```python
from build123d import *

# Parameters (mm, degrees)
SKETCH1_W            = 93
SKETCH1_H            = 60
BOSS_EXTRUDE1_DEPTH  = 3
SKETCH2_W            = 3
SKETCH2_H            = 5
CUT_EXTRUDE1_DEPTH   = 3
SKETCH4_W            = 35
SKETCH4_H            = 3
BOSS_EXTRUDE2_DEPTH  = 45
FILLET1_R            = 5
SKETCH5_W            = 3
SKETCH5_H            = 5
CUT_EXTRUDE3_DEPTH   = 4
LPATTERN1_COUNT      = 4
LPATTERN1_PITCH      = 30
LPATTERN1_COUNT_DIR2 = 2
LPATTERN1_PITCH_DIR2 = 30
SKETCH6_R            = 2
CUT_EXTRUDE4_DEPTH   = 4
SKETCH7_W            = 3
SKETCH7_H            = 5
CUT_EXTRUDE5_DEPTH   = 4
SKETCH8_R            = 3
CUT_EXTRUDE6_DEPTH   = 4


with BuildPart() as part:
    # Sketch1 → Boss-Extrude1 (new body)
    with BuildSketch(Plane(origin=(0, 0, 0), x_dir=(1, 0, 0), z_dir=(0, 1, 0))):
        with Locations((46.5, 30)):
            Rectangle(SKETCH1_W, SKETCH1_H)
    extrude(amount=BOSS_EXTRUDE1_DEPTH)

    # Sketch2 → Cut-Extrude1 (cut)
    with BuildSketch(Plane(origin=(0, 3, 0), x_dir=(1, 0, 0), z_dir=(0, 1, 0))):
        with Locations((63.5, 12.5)):
            Rectangle(SKETCH2_W, SKETCH2_H)
        with Locations((47.5, 12.5)):
            Rectangle(SKETCH2_W, SKETCH2_H)
        with Locations((29.5, 12.5)):
            Rectangle(SKETCH2_W, SKETCH2_H)
        with Locations((6.5, 12.5)):
            Rectangle(SKETCH2_W, SKETCH2_H)
    cut_extrude1 = extrude(amount=-CUT_EXTRUDE1_DEPTH, mode=Mode.SUBTRACT)

    # Mirror1: Cut-Extrude1 across plane
    add(cut_extrude1.mirror(Plane.XY.offset(-30)), mode=Mode.SUBTRACT)

    # Sketch4 → Boss-Extrude2 (add)
    with BuildSketch(Plane(origin=(0, 0, -60), x_dir=(-1, 0, 0), z_dir=(0, 0, -1))):
        with Locations((-75.5, 1.5)):
            Rectangle(SKETCH4_W, SKETCH4_H)
    extrude(amount=BOSS_EXTRUDE2_DEPTH)

    # Fillet1
    fillet1_edges = [part.edges().sort_by_distance(p)[0] for p in [
        (58, 1.5, -60),
        (93, 1.5, -105),
        (58, 1.5, -105),
        (0, 1.5, -60),
        (93, 1.5, 0),
        (0, 1.5, 0),
    ]]
    fillet(fillet1_edges, radius=FILLET1_R)

    # Sketch5 → Cut-Extrude3 (cut, through all)
    with BuildSketch(Plane(origin=(0, 3, 0), x_dir=(1, 0, 0), z_dir=(0, 1, 0))):
        with Locations((86.5, 7.5)):
            Rectangle(SKETCH5_W, SKETCH5_H)
        with Locations((79.5, 7.5)):
            Rectangle(SKETCH5_W, SKETCH5_H)
    cut_extrude3 = extrude(amount=-CUT_EXTRUDE3_DEPTH, mode=Mode.SUBTRACT)

    # LPattern1: Cut-Extrude3 4 × 2
    with Locations(*[(j * LPATTERN1_PITCH_DIR2, 0, -i * LPATTERN1_PITCH) for i in range(LPATTERN1_COUNT) for j in range(LPATTERN1_COUNT_DIR2) if (i, j) != (0, 0)]):
        add(cut_extrude3, mode=Mode.SUBTRACT)

    # Sketch6 → Cut-Extrude4 (cut, through all)
    with BuildSketch(Plane(origin=(0, 3, 0), x_dir=(1, 0, 0), z_dir=(0, 1, 0))):
        with Locations((18, 14)):
            Circle(SKETCH6_R)
        with Locations((18, 46)):
            Circle(SKETCH6_R)
        with Locations((55.5, 50.5)):
            Circle(SKETCH6_R)
        with Locations((55.5, 9.5)):
            Circle(SKETCH6_R)
        with Locations((72, 9.5)):
            Circle(SKETCH6_R)
        with Locations((72, 50.5)):
            Circle(SKETCH6_R)
        with Locations((72, 85.5)):
            Circle(SKETCH6_R)
    extrude(amount=-CUT_EXTRUDE4_DEPTH, mode=Mode.SUBTRACT)

    # Sketch7 → Cut-Extrude5 (cut, through all)
    with BuildSketch(Plane(origin=(0, 3, 0), x_dir=(1, 0, 0), z_dir=(0, 1, 0))):
        with Locations((63.5, 67.5)):
            Rectangle(SKETCH7_W, SKETCH7_H)
        with Locations((63.5, 97.5)):
            Rectangle(SKETCH7_W, SKETCH7_H)
    extrude(amount=-CUT_EXTRUDE5_DEPTH, mode=Mode.SUBTRACT)

    # Sketch8 → Cut-Extrude6 (cut, through all)
    with BuildSketch(Plane(origin=(0, 3, 0), x_dir=(1, 0, 0), z_dir=(0, 1, 0))):
        with Locations((35, 12.5)):
            Circle(SKETCH8_R)
        with Locations((35, 47.5)):
            Circle(SKETCH8_R)
    extrude(amount=-CUT_EXTRUDE6_DEPTH, mode=Mode.SUBTRACT)


solid = part.part
```
Could you check a few things on this model? Use its own coordinates, in mm. Round coordinates to 2 decimals unless told otherwise and drop trailing zeros. Loops run counter-clockwise (first coordinate to the right, second up) from the corner with the lowest first, then second, coordinate; pieces in that order, holes last.
Q1. I want a section at A-A (x = 18). Write out the boundary of the cut face in (y, z), and give its area (3 significant figures).
Q2. For P1, Ø0.9, axis at x = 29.5, y = 1.5, coming from the -Z side, with a flat end and sliding along its axis, tell me the tip position at first contact or that it passes through.
Q3. I want a section at C-C (x = 72). Write out the boundary of the cut face in (y, z).
Q4. Please list where these lines run through material, in increasing order: L1, parallel to Z at x = 35, y = 1.1; L2, parallel to Z at x = 87.5, y = 2.3; L3, parallel to X at y = 2.85, z = -99.
Q5. I want a section at B-B (z = -97.5). Write out the boundary of the cut face in (x, y), and give its area (3 significant figures).
Q6. Thinking about a two-plate mould opening in Z: for faces 1 (the flat face through (29, 1, -60)), 2 (the flat face through (63, 2, -70)), which applies, pulls with the +Z half, pulls with the -Z half, needs draft (parallel to the pull), parting line crosses it, or undercut?
Q7. I want a section at D-D (x = 35). Write out the boundary of the cut face in (y, z).
Answer below:
1. outline: (0, -60) - (3, -60) - (3, -48) - (0, -48) - close; (0, -44) - (3, -44) - (3, -16) - (0, -16) - close; (0, -12) - (3, -12) - (3, 0) - (0, 0) - close
1. area: 156 mm2
2. P1: stops at z = -60
3. outline: (0, -105) - (3, -105) - (3, -87.5) - (0, -87.5) - close; (0, -83.5) - (3, -83.5) - (3, -52.5) - (0, -52.5) - close; (0, -48.5) - (3, -48.5) - (3, -11.5) - (0, -11.5) - close; (0, -7.5) - (3, -7.5) - (3, 0) - (0, 0) - close
4. L1: z = -60 to -50.5, -44.5 to -15.5, -9.5 to 0
4. L2: z = -105 to -100, -95 to -70, -65 to -40, -35 to -10, -5 to 0
4. L3: x = 58 to 62, 65 to 78, 81 to 85, 88 to 93
5. outline: (58, 0) - (62, 0) - (62, 3) - (58, 3) - close; (65, 0) - (78, 0) - (78, 3) - (65, 3) - close; (81, 0) - (85, 0) - (85, 3) - (81, 3) - close; (88, 0) - (93, 0) - (93, 3) - (88, 3) - close
5. area: 78.0 mm2
6. face 1: pulls with the -Z half
6. face 2: undercut
7. outline: (0, -60) - (3, -60) - (3, -50.5) - (0, -50.5) - close; (0, -44.5) - (3, -44.5) - (3, -15.5) - (0, -15.5) - close; (0, -9.5) - (3, -9.5) - (3, 0) - (0, 0) - close
